The figure shows three views and two pictorial views of one solid part (mm, origin at its lowest corner). Answer the questions. A direction names the side the tool comes from. Round coordinates to 2 decimals unless told otherwise and drop trailing zeros. Order: outer loops, then holes, each group sorted by start corner. A loop starts at its lowest first (then second) coordinate and runs counter-clockwise, first axis right, second up.
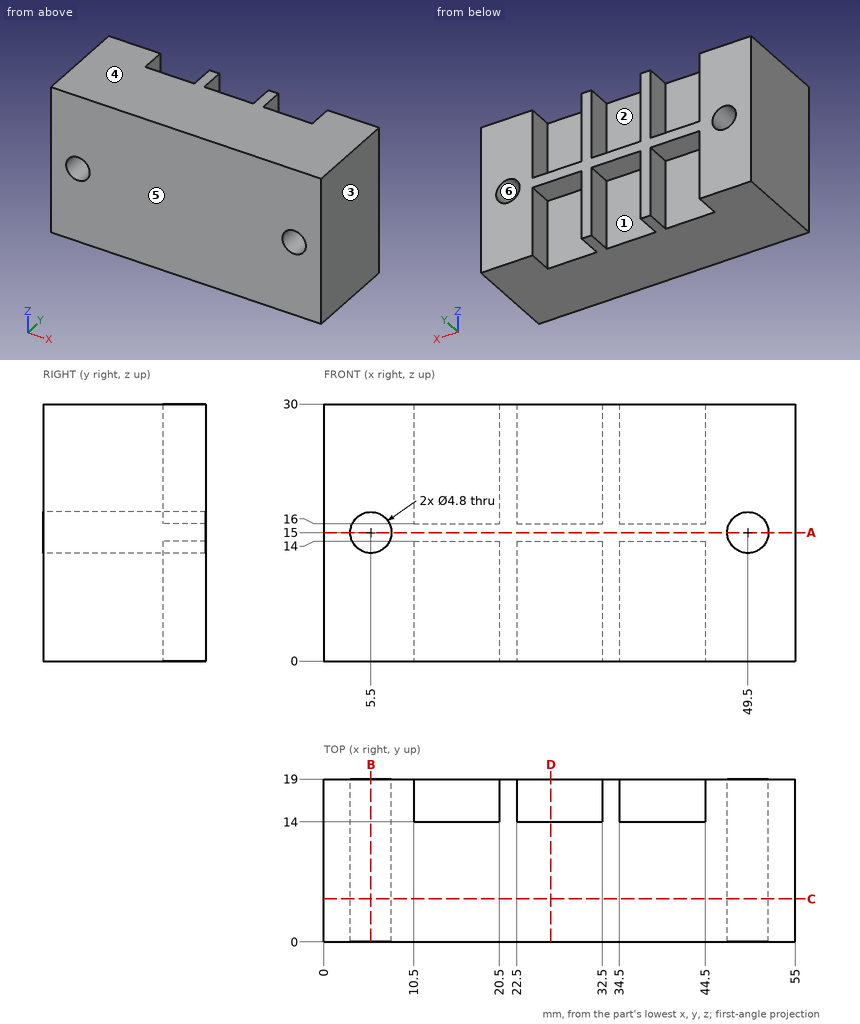
Item 1: Find section D-D (x = 26.5). Write down the section's boundary in (y, z), plus the area to 3 significant figures.
Item 2: Find section C-C (y = 5). Write down the section's boundary in (x, z).
Item 3: A tool of negligible diameter and unlimited length cuts with its end or side. For the marked faces 1, 2 and 3, from which of +Z, -Z, +X, -X, +Y, -Y can it reach the whole face along a straight path? Write none if from no direction.
Item 4: Find section B-B (x = 5.5). Write down the section's boundary in (y, z), plus the area to 3 significant figures.
Item 5: Find section A-A (z = 15). Write down the section's boundary in (x, y).
Item 6: For a pull along Z with two mould halves and no side action, classify the marked faces 4, 5 and 6 as released by +Z, released by -Z, zero draft, split by the parting line, or undercut.
Item 7: Find the intervals of material crossed by line 1 along X through (y, z) = (5, 15); line 2 along X through (y, z) = (1, 13.5); line 3 along Z through (x, y) = (49.5, 14.5), in increasing order.
Item 8: Given pin 1 (1.5 mm diameter, centred on x = 37.5, y = 17, fed in from -Z); pin 2 (3 mm diameter, centred on x = 26, z = 7, fed in from +Y), each flat-ended and moving along its own axis, determine where each tip first touches the part or whether it passes through.
Model answer:
1. outline: (0, 0) - (14, 0) - (14, 14) - (19, 14) - (19, 16) - (14, 16) - (14, 30) - (0, 30) - close
1. area: 430 mm2
2. outline: (0, 0) - (55, 0) - (55, 30) - (0, 30) - close; hole circle Ø4.8 at (5.5, 15); hole circle Ø4.8 at (49.5, 15)
3. face 1: -Z, +Y
3. face 2: +Z, +Y
3. face 3: +Z, -Z, +X, +Y, -Y
4. outline: (0, 0) - (19, 0) - (19, 12.6) - (0, 12.6) - close; (0, 17.4) - (19, 17.4) - (19, 30) - (0, 30) - close
4. area: 479 mm2
5. outline: (0, 0) - (3.1, 0) - (3.1, 19) - (0, 19) - close; (7.9, 0) - (47.1, 0) - (47.1, 19) - (7.9, 19) - close; (51.9, 0) - (55, 0) - (55, 19) - (51.9, 19) - close
6. face 4: released by +Z
6. face 5: zero draft
6. face 6: undercut
7. line 1: x = 0 to 3.1, 7.9 to 47.1, 51.9 to 55
7. line 2: x = 0 to 3.63, 7.37 to 47.63, 51.37 to 55
7. line 3: z = 0 to 12.6, 17.4 to 30
8. pin 1: stops at z = 14
8. pin 2: stops at y = 14
